Design review of the part built by this model. Coordinates are the model's own, in mm. A direction names the side the tool comes from. Give positions to 0.01 mm unless a question says otherwise; leave off trailing zeros. Order: outer loops, then holes, each group sorted by start corner. A loop starts at its lowest first (then second) coordinate and runs counter-clockwise, first axis right, second up. Notation, with made-up numbers: (2.25, 40.5) - (16.25, 40.5) arc R19 ccw to (16.25, 77.5) - close; hole circle Ø1 at (66, 26). An arc over 180 degrees is marked (long way). Write each question's results on one line, items separated by ' | '. Start each with the question number.
```python
from build123d import *

# Parameters (mm, degrees)
F0_W      = 50
F0_H      = 50
F1_DEPTH  = 4
F2_W      = 43.4
F2_H      = 43.4
F3_DEPTH  = 3
F4_R      = 3
F5_DEPTH  = 25
F6_R      = 5
F6_R_2    = 3
F7_DEPTH  = 3
F8_R      = 16
F9_DEPTH  = 5
F10_R     = 11
F11_DEPTH = 25
F12_R     = 3


# Not quite as in the source:
# - a feature names something its author has since deleted; it is built from what else it names


with BuildPart() as f1:
    # F0 (on Front) → F1 (new body)
    with BuildSketch(Plane.XZ):
        Rectangle(F0_W, F0_H)
    extrude(amount=-F1_DEPTH)

    # F2 (on face) → F3 (join)
    with BuildSketch(Plane(origin=(0, 4, 0), x_dir=(-1, 0, 0), z_dir=(0, 1, 0))):
        Rectangle(F2_W, F2_H)
    extrude(amount=F3_DEPTH)

    # F4 (on face) → F5 (cut)
    with BuildSketch(Plane(origin=(0, 7, 0), x_dir=(-1, 0, 0), z_dir=(0, 1, 0))):
        with Locations((-16.5, 16.5)):
            Circle(F4_R)
        with Locations((16.5, 16.5)):
            Circle(F4_R)
        with Locations((16.5, -16.5)):
            Circle(F4_R)
        with Locations((-16.5, -16.5)):
            Circle(F4_R)
    extrude(amount=-F5_DEPTH, mode=Mode.SUBTRACT)

    # F6 (on face) → F7 (cut)
    with BuildSketch(Plane.XZ):
        with Locations((-16.5, 16.5)):
            Circle(F6_R)
        with Locations((-16.5, 16.5)):
            Circle(F6_R_2, mode=Mode.SUBTRACT)
        with Locations((16.5, 16.5)):
            Circle(F6_R)
        with Locations((16.5, 16.5)):
            Circle(F6_R_2, mode=Mode.SUBTRACT)
        with Locations((16.5, -16.5)):
            Circle(F6_R)
        with Locations((16.5, -16.5)):
            Circle(F6_R_2, mode=Mode.SUBTRACT)
        with Locations((-16.5, -16.5)):
            Circle(F6_R)
        with Locations((-16.5, -16.5)):
            Circle(F6_R_2, mode=Mode.SUBTRACT)
    extrude(amount=-F7_DEPTH, mode=Mode.SUBTRACT)

    # F8 (on face) → F9 (cut)
    with BuildSketch(Plane(origin=(0, 7, 0), x_dir=(-1, 0, 0), z_dir=(0, 1, 0))):
        Circle(F8_R)
    extrude(amount=-F9_DEPTH, mode=Mode.SUBTRACT)

    # F10 (on face) → F11 (cut)
    with BuildSketch(Plane.XZ):
        Circle(F10_R)
    extrude(amount=-F11_DEPTH, mode=Mode.SUBTRACT)

    # F12
    f12_edges = [f1.edges().sort_by_distance(p)[0] for p in [
        (21.7, 5.5, 21.7),
        (-21.7, 5.5, 21.7),
        (-21.7, 5.5, -21.7),
        (21.7, 5.5, -21.7),
    ]]
    fillet(f12_edges, radius=F12_R)


solid = f1.part
```
Q1. For line 1 (Z direction, x = -16.5, y = 0.7); line 2 (Z direction, x = 16.5, y = 4.3); line 3 (X direction, y = 6.5, z = -14), list the stretches that pass through material, from the lowest coordinate up. Write a range as [from, to].
Q2. Add section C-C (x = 0). Give the boundary of the cut face in (y, z), plus the area to 3 significant figures.
Q3. Machinability: for faces 4 (the flat face through (0, 5, 21.7)), 5 (the flat face through (-3, 2, 11)), 6 (the cylindrical face through (20.84, 5.52, -20.8)), 7 (the flat face through (21.7, 5, 0)), 8 (the flat face through (-14, 3, -19)), which of the approach directions +Z, -Z, +X, -X, +Y, -Y give a long, thin tool a straight path to every point of the face, cutting with its end or side? Answer none if there is none.
Q4. Draft analysis for pull direction Z (two halves, no side actions). For faces 1 (the cylindrical face through (-15.85, 5.03, -19.43)), 2 (the flat face through (-23, 4, 0)), 3 (the cylindrical face through (-20.84, 5.52, -20.8)), state which applies: pulls with the +Z half, pulls with the -Z half, needs draft (parallel to the pull), parting line crosses it, or undercut.
Q5. Insertion check: pin 1 Ø3 at (x, z) = (17.5, -14) entering from -Y; pin 2 Ø1 at (x, z) = (-9, -11.5) entering from +Y; pin 3 Ø0.9 at (x, y) = (6.5, 6) entering from +Z. Each pin has a flat end and moves straight along its axis. Give the tip position at first contact, or say it passes through.
Q6. Add section D-D (z = 15). Give the boundary of the cut face in (x, y).
Q7. Add section A-A (y = 5). Give the boundary of the cut face in (x, z).
Q8. Add section B-B (z = 0). Give the boundary of the cut face in (x, y).
Verdict:
1) line 1: z = [-25, -21.5], [-11.5, 11.5], [21.5, 25] | line 2: z = [-21.7, -19.5], [-13.5, 13.5], [19.5, 21.7] | line 3: x = [-21.7, -18.16], [-14.84, -7.75], [7.75, 14.84], [18.16, 21.7]
2) outline: (0, -25) - (4, -25) - (4, -21.7) - (7, -21.7) - (7, -16) - (2, -16) - (2, -11) - (0, -11) - close; (0, 11) - (2, 11) - (2, 16) - (7, 16) - (7, 21.7) - (4, 21.7) - (4, 25) - (0, 25) - close | area: 126 mm2
3) face 4: +Z, +X, -X, +Y | face 5: +Y | face 6: -Z, +X, +Y | face 7: +Z, -Z, +X, +Y | face 8: -Y
4) face 1: undercut | face 2: needs draft | face 3: pulls with the -Z half
5) pin 1: stops at y = 3 | pin 2: stops at y = 2 | pin 3: stops at z = 21.7
6) outline: (-25, 0) - (-21.27, 0) - (-21.27, 3) - (-19.1, 3) - (-19.1, 7) - (-21.7, 7) - (-21.7, 4) - (-25, 4) - close; (-13.9, 3) - (-11.73, 3) - (-11.73, 0) - (11.73, 0) - (11.73, 3) - (13.9, 3) - (13.9, 7) - (5.57, 7) - (5.57, 2) - (-5.57, 2) - (-5.57, 7) - (-13.9, 7) - close; (19.1, 3) - (21.27, 3) - (21.27, 0) - (25, 0) - (25, 4) - (21.7, 4) - (21.7, 7) - (19.1, 7) - close
7) outline: (-21.7, -18.7) arc R3 ccw to (-18.7, -21.7) - (18.7, -21.7) arc R3 ccw to (21.7, -18.7) - (21.7, 18.7) arc R3 ccw to (18.7, 21.7) - (-18.7, 21.7) arc R3 ccw to (-21.7, 18.7) - close; hole circle Ø6 at (-16.5, -16.5); hole circle Ø6 at (-16.5, 16.5); hole circle Ø32 at (0, 0); hole circle Ø6 at (16.5, -16.5); hole circle Ø6 at (16.5, 16.5)
8) outline: (-25, 0) - (-11, 0) - (-11, 2) - (-16, 2) - (-16, 7) - (-21.7, 7) - (-21.7, 4) - (-25, 4) - close; (11, 0) - (25, 0) - (25, 4) - (21.7, 4) - (21.7, 7) - (16, 7) - (16, 2) - (11, 2) - close
